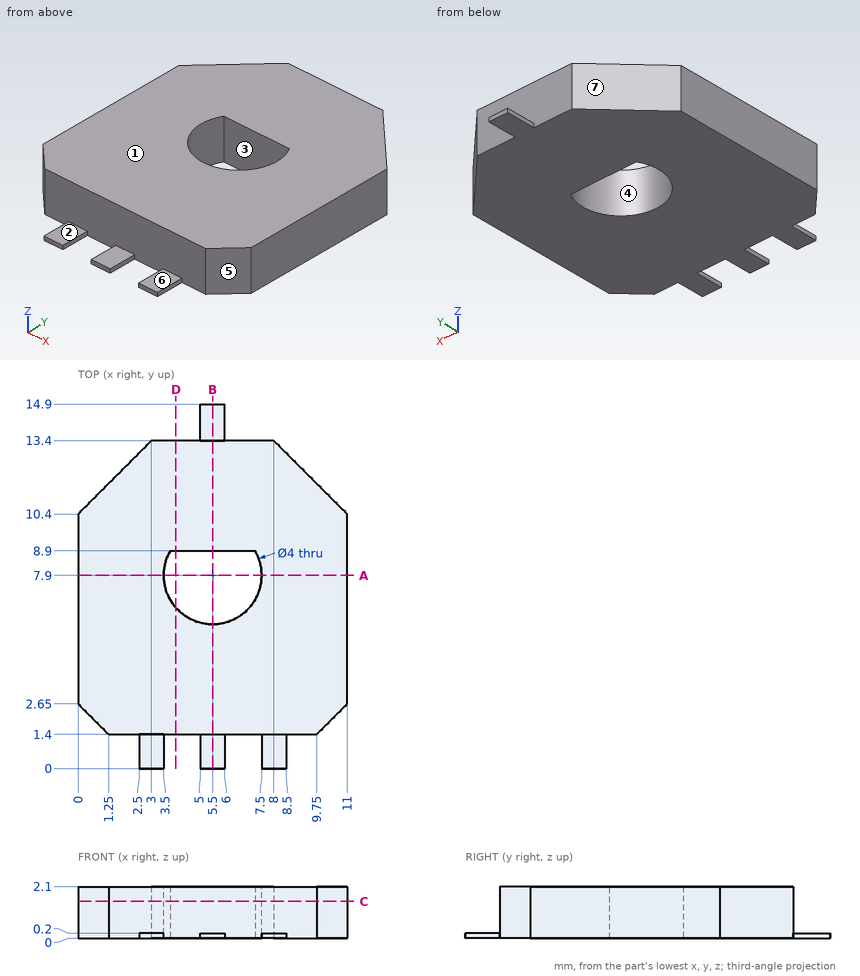
Job drawing, mm, ordinate dimensions from the low corner. One solid piece. A direction names the side the tool comes from. Coordinates: 2 decimals unless noted, no trailing zeros. Order: outer loops, then holes, each group sorted by start corner. A loop starts at its lowest first (then second) coordinate and runs counter-clockwise, first axis right, second up. Notation, with made-up numbers: M -27.75,16 L 9.25,16 A14 cw 9.25,25 Z; hole C 68.25,43.25 d5. An arc over 180 degrees is marked long. Answer as CSV lines item,"result".
(1) Band-saw the part on D-D, the plane x = 4. List the corners of the cut face in (y, z).
Geometry says:
outline,"M 1.4,0 L 6.58,0 L 6.58,2.1 L 1.4,2.1 Z; M 8.9,0 L 13.4,0 L 13.4,2.1 L 8.9,2.1 Z"
(2) Band-saw the part on A-A, the plane y = 7.9. List the corners of the cut face in (x, z).
Geometry says:
outline,"M 0,0 L 3.5,0 L 3.5,2.1 L 0,2.1 Z; M 7.5,0 L 11,0 L 11,2.1 L 7.5,2.1 Z"
(3) 3-axis set-ups, long thin cutter, end or side, ignore diameter. For the marked faces 1, 2 and 3: which of +Z, -Z, +X, -X, +Y, -Y reach the whole face in a straight line?
Geometry says:
face 1,"+Z, +X, -X, +Y, -Y"
face 2,"+Z, +X, -X, -Y"
face 3,"+Z, -Z"
(4) Band-saw the part on C-C, the plane z = 1.5. List the corners of the cut face in (x, y).
Geometry says:
outline,"M 0,2.65 L 1.25,1.4 L 9.75,1.4 L 11,2.65 L 11,10.4 L 8,13.4 L 3,13.4 L 0,10.4 Z; hole M 3.77,8.9 A2 ccw long 7.23,8.9 Z"
(5) Flat gauge pins, fed straight in: pin 1 (0.5 mm diameter, centred on x = 5.5, y = 1, fed in from +Z); pin 2 (1 mm diameter, centred on x = 6, z = 1, fed in from -Y). Where does each tip first touch, or does it go through?
Geometry says:
pin 1,"stops at z = 0.2"
pin 2,"stops at y = 1.4"
(6) Band-saw the part on B-B, the plane x = 5.5. List the corners of the cut face in (y, z), then the cut area to 3 significant figures.
Geometry says:
outline,"M 0,0 L 5.9,0 L 5.9,2.1 L 1.4,2.1 L 1.4,0.2 L 0,0.2 Z; M 8.9,0 L 14.9,0 L 14.9,0.2 L 13.4,0.2 L 13.4,2.1 L 8.9,2.1 Z"
area,"19.5 mm2"
(7) Wall check: line 1 along X through (y, z) = (7.9, 0.5); line 2 along Y through (x, z) = (5.5, 0.4); line 3 along Y through (x, z) = (9, 0.3). Give the ranges that are in metal, low to high.
Geometry says:
line 1,"x = 0 to 3.5, 7.5 to 11"
line 2,"y = 1.4 to 5.9, 8.9 to 13.4"
line 3,"y = 1.4 to 12.4"
(8) Pull direction Y, two halves, no side cores. Call the marked faces 4, 5, 6 and 7: +Y half, -Y half, draft (parallel to the pull), parting line (faces both ways), or undercut.
Geometry says:
face 4,"undercut"
face 5,"-Y half"
face 6,"draft"
face 7,"+Y half"
